The drawing under review shows one solid part. Ordinate dimensions are in mm from its lowest x, y, z. A direction names the side the tool comes from. Give positions to 0.01 mm unless a question says otherwise; leave off trailing zeros. Write each loop counter-clockwise with the first axis right and the second up, starting at its lowest first coordinate (ties: lowest second). Pieces come first, ordered by that corner, then holes.
Q1. Machinability: for the marked faces 4, 5 and 6, which of the approach directions +Z, -Z, +X, -X, +Y, -Y give a long, thin tool a straight path to every point of the face, cutting with its end or side? Answer none if there is none.
Q2. We need section A-A (z = 12.7). Write out the cut boundary in (x, y) (1 decimal), then the cut area to 3 significant figures.
Q3. Insertion check: P1, Ø2.5, axis at x = 28, z = 5.5, coming from the +Y side (1 decimal); P2, Ø4, axis at x = 3.81, z = 12.7, coming from the +Y side (1 decimal); P3, Ø2, axis at x = 17, y = 5, coming from the +Z side (3 decimals). Each pin has a flat end and moves straight along its axis. Give the tip position at first contact, or say it passes through.
Q4. Mouldability with a two-part tool opening along X and no side actions: class the marked faces 1, 2 and 3 as released by +X, released by -X, zero draft, split by the parting line, or undercut.
Q5. We need section C-C (y = 1). Write out the cut boundary in (x, z) (1 decimal), then the cut area to 3 significant figures.
Q6. For line 1 (X direction, y = 0.7, z = 12.7); line 2 (Y direction, x = 25, z = 9.25) (1 decimal); line 3 (Z direction, x = 21, y = 4.25) (1 decimal), list the stretches that pass through material, from the lowest coordinate up.
Q7. We need section B-B (x = 17.5). Write out the cut boundary in (y, z) (1 decimal).
Q8. We need section D-D (y = 2.75). Write out the cut boundary in (x, z) (1 decimal).
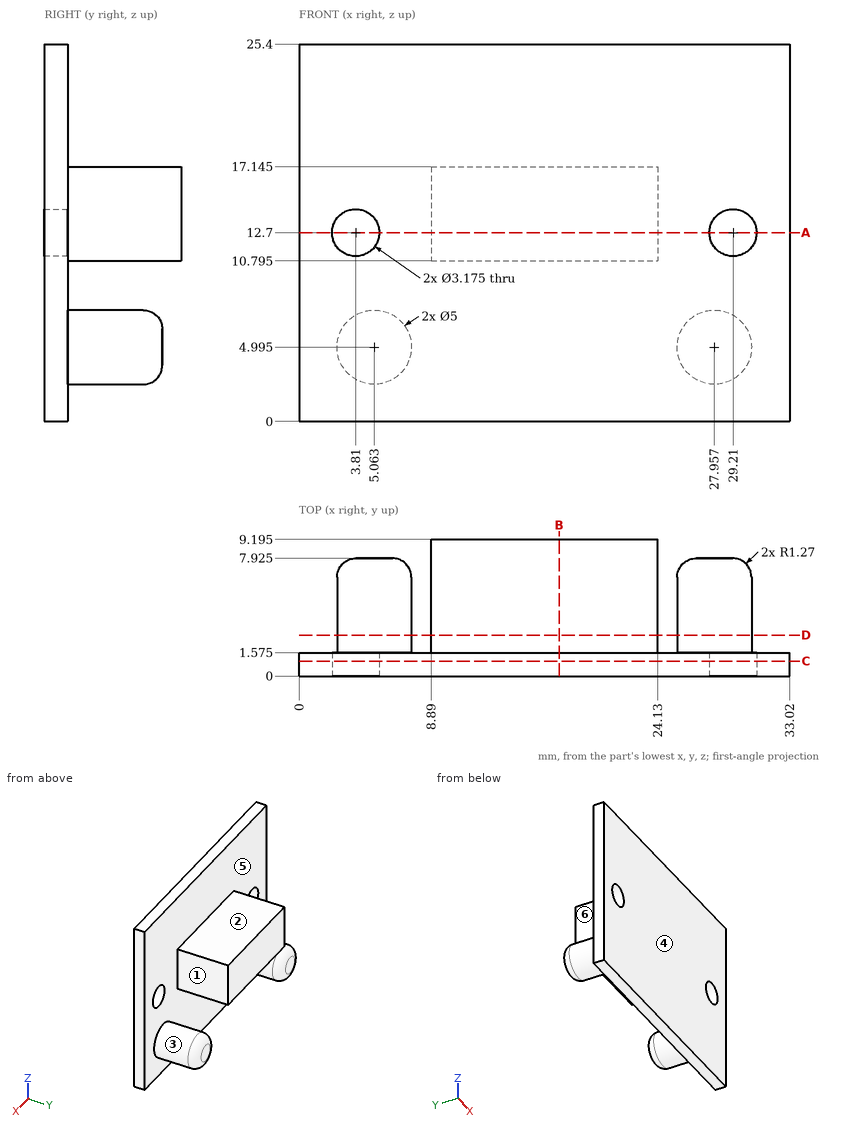
Computed:
1. face 4: +Z, -Z, +X, -X, -Y
1. face 5: +Y
1. face 6: +Z, -Z, -X, +Y
2. outline: (0, 0) - (2.2, 0) - (2.2, 1.6) - (0, 1.6) - close; (5.4, 0) - (27.6, 0) - (27.6, 1.6) - (24.1, 1.6) - (24.1, 9.2) - (8.9, 9.2) - (8.9, 1.6) - (5.4, 1.6) - close; (30.8, 0) - (33, 0) - (33, 1.6) - (30.8, 1.6) - close
2. area: 158 mm2
3. P1: stops at y = 7.9
3. P2: stops at y = 1.6
3. P3: stops at z = 17.145
4. face 1: released by +X
4. face 2: zero draft
4. face 3: undercut
5. outline: (0, 0) - (33, 0) - (33, 25.4) - (0, 25.4) - close; hole circle Ø3.2 at (3.8, 12.7); hole circle Ø3.2 at (29.2, 12.7)
5. area: 823 mm2
6. line 1: x = 0 to 2.22, 5.4 to 27.62, 30.8 to 33.02
6. line 2: y = 0 to 1.6
6. line 3: z = 10.8 to 17.1
7. outline: (0, 0) - (1.6, 0) - (1.6, 10.8) - (9.2, 10.8) - (9.2, 17.1) - (1.6, 17.1) - (1.6, 25.4) - (0, 25.4) - close
8. outline: circle Ø5 at (5.1, 5); (8.9, 10.8) - (24.1, 10.8) - (24.1, 17.1) - (8.9, 17.1) - close; circle Ø5 at (28, 5)
